from build123d import *

# Parameters (mm, degrees)
F0_R      = 1.5
F0_R_2    = 4.25
F1_DEPTH  = 3
F2_DEPTH  = 22
F3_W      = 9.5
F3_H      = 11
F2_FACE_W = 100
F2_FACE_H = 22
F4_DEPTH  = 50.001
F5_W      = 17
F5_H      = 3.3289747284
F6_DEPTH  = 76.9
F7_W      = 12.5
F7_H      = 8.2103219628
F7_H_2    = 8.3398447186
F7_H_3    = 8.5524427253
F8_DEPTH  = 63.2
F9_R      = 2
F10_DEPTH = 67.3


# Not quite as in the source:
# - a feature of the source that left no trace in its solid (it failed there, or was rolled back) is left out


with BuildPart() as f1:
    # F0 (on Top) → F1 (new body)
    with BuildSketch(Plane.XY):
        with BuildLine():
            Line((-48.5, -48.5), (0, -48.5))
            Line((0, -48.5), (0, -35.75))
            ThreePointArc((0, -35.75), (-4.25, -31.5), (0, -27.25))
            Line((0, -27.25), (0, -11.75))
            ThreePointArc((0, -11.75), (-4.25, -7.5), (0, -3.25))
            Line((0, -3.25), (0, 10.5))
            Line((0, 10.5), (-32, 10.5))
            Line((-32, 10.5), (-32, 26.5))
            Line((-32, 26.5), (0, 26.5))
            Line((0, 26.5), (0, 48.5))
            Line((0, 48.5), (-48.5, 48.5))
            Line((-48.5, 48.5), (-48.5, -48.5))
        make_face()
        with Locations((-32.5, -20.5)):
            Circle(F0_R, mode=Mode.SUBTRACT)
        with Locations((-32.5, -11.5)):
            Circle(F0_R, mode=Mode.SUBTRACT)
        with Locations((-32.5, -2.5)):
            Circle(F0_R, mode=Mode.SUBTRACT)
        with Locations((-14, -19.5)):
            Circle(F0_R_2, mode=Mode.SUBTRACT)
        with BuildLine():
            Line((0, -35.75), (0, -48.5))
            Line((0, -48.5), (48.5, -48.5))
            Line((48.5, -48.5), (48.5, 48.5))
            Line((48.5, 48.5), (0, 48.5))
            Line((0, 48.5), (0, 26.5))
            Line((0, 26.5), (32, 26.5))
            Line((32, 26.5), (32, 10.5))
            Line((32, 10.5), (0, 10.5))
            Line((0, 10.5), (0, -3.25))
            ThreePointArc((0, -3.25), (3.00520382, -4.49479618), (4.25, -7.5))
            ThreePointArc((4.25, -7.5), (3.00520382, -10.50520382), (0, -11.75))
            Line((0, -11.75), (0, -27.25))
            ThreePointArc((0, -27.25), (3.00520382, -28.49479618), (4.25, -31.5))
            ThreePointArc((4.25, -31.5), (3.00520382, -34.50520382), (0, -35.75))
        make_face()
        with Locations((14, -19.5)):
            Circle(F0_R_2, mode=Mode.SUBTRACT)
    extrude(amount=F1_DEPTH)

    # F0 (on Top) → F2 (join)
    with BuildSketch(Plane.XY):
        Polygon((50, 50), (-50, 50), (-50, -50), (0, -50), (50, -50), align=None)
        Polygon((48.5, -48.5), (0, -48.5), (-48.5, -48.5), (-48.5, 48.5), (0, 48.5), (48.5, 48.5), align=None, mode=Mode.SUBTRACT)
    extrude(amount=F2_DEPTH)

    # F3 (on Right) + F2_face (on face) → F4 (cut, through all)
    with BuildSketch(Plane.YZ):
        with Locations((-41.75, 25.5)):
            Rectangle(F3_W, F3_H)
    with BuildSketch(Plane(origin=(50, 0, 11), x_dir=(0, 1, 0), z_dir=(1, 0, 0))):
        Rectangle(F2_FACE_W, F2_FACE_H)
    extrude(amount=F4_DEPTH, mode=Mode.SUBTRACT)

    # F5 (on Right) → F6 (cut)
    with BuildSketch(Plane.YZ):
        with Locations((-22, 21.6644873642)):
            Rectangle(F5_W, F5_H)
    extrude(amount=F6_DEPTH, mode=Mode.SUBTRACT)

    # F7 (on Right) → F8 (cut)
    with BuildSketch(Plane.YZ):
        with Locations((32.75, 21.6051609814)):
            Rectangle(F7_W, F7_H)
        with Locations((15.25, 21.6699223593)):
            Rectangle(F7_W, F7_H_2)
        with Locations((-2.25, 21.7762213627)):
            Rectangle(F7_W, F7_H_3)
    extrude(amount=F8_DEPTH, mode=Mode.SUBTRACT)

    # F9 (on Right) → F10 (cut)
    with BuildSketch(Plane.YZ):
        with Locations((-12, 22)):
            Circle(F9_R)
        with Locations((-4, 22)):
            Circle(F9_R)
        with Locations((-20, 22)):
            Circle(F9_R)
        with Locations((-35.5, 22)):
            Circle(F9_R)
    extrude(amount=-F10_DEPTH, mode=Mode.SUBTRACT)


solid = f1.part
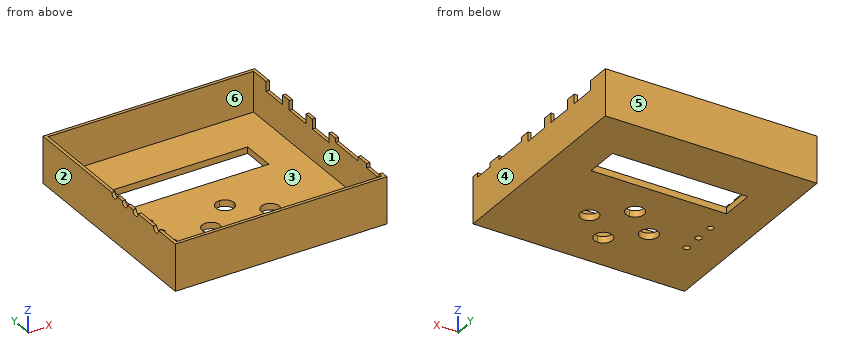
Model file for the job. Use its own axes, mm. Face numbers are marked on the shaded views. A direction names the side the tool comes from. Give positions to 0.01 mm unless a question says otherwise; leave off trailing zeros. Order: outer loops, then holes, each group sorted by start corner. A loop starts at its lowest first (then second) coordinate and runs counter-clockwise, first axis right, second up. Notation, with made-up numbers: (-10.5, 81) -> (27.5, 81) arc R20 cw to (27.5, 107) -> close; hole circle Ø8 at (0, 15.5). An arc over 180 degrees is marked (long way). Use CSV: the item, a comma, the result in double quotes.
1. Mould opens along X. For the marked faces 3, 4, 5 and 6 say: +X half, -X half, draft (parallel to the pull), parting line (faces both ways), or undercut.
Outcome:
face 3,"undercut"
face 4,"+X half"
face 5,"draft"
face 6,"undercut"
2. Band-saw the part on C-C, the plane y = 14. Give the cut face in (x, z).
Outcome:
outline,"(-50, 0) -> (-32, 0) -> (-32, 3) -> (-48.5, 3) -> (-48.5, 22) -> (-50, 22) -> close; (32, 0) -> (50, 0) -> (50, 17.5) -> (48.5, 17.5) -> (48.5, 3) -> (32, 3) -> close"
3. 3-axis set-ups, long thin cutter, end or side, ignore diameter. For the marked faces 1 and 2: which of +Z, -Z, +X, -X, +Y, -Y reach the whole face in a straight line?
Outcome:
face 1,"+Z"
face 2,"+Z, -Z, -X, +Y, -Y"
4. Band-saw the part on A-A, the plane x = -12. Give the cut face in (y, z).
Outcome:
outline,"(-50, 0) -> (-23.25, 0) -> (-23.25, 3) -> (-48.5, 3) -> (-48.5, 22) -> (-50, 22) -> close; (-15.75, 0) -> (10.5, 0) -> (10.5, 3) -> (-15.75, 3) -> close; (26.5, 0) -> (50, 0) -> (50, 22) -> (48.5, 22) -> (48.5, 3) -> (26.5, 3) -> close"
5. Drop flat-ended pins along their axis: pin 1 (0.8 mm diameter, centred on x = 49.5, y = -22, fed in from +Z); pin 2 (2.5 mm diameter, centred on x = -32.5, y = -11.5, fed in from -Z); pin 3 (1.2 mm diameter, centred on x = 49, y = -2.5, fed in from +Z); pin 4 (4 mm diameter, centred on x = -32.5, y = -20.5, fed in from +Z). Give the stop position or say it passes through.
Outcome:
pin 1,"z = 20"
pin 2,"through"
pin 3,"z = 17.5"
pin 4,"z = 3"
6. Band-saw the part on B-B, the plane z = 6.5. Give the cut face in (x, y).
Outcome:
outline,"(-50, -50) -> (50, -50) -> (50, 50) -> (-50, 50) -> close; hole (-48.5, -48.5) -> (48.5, -48.5) -> (48.5, 48.5) -> (-48.5, 48.5) -> close"
7. Band-saw the part on D-D, the plane x = 26. Give the cut face in (y, z).
Outcome:
outline,"(-50, 0) -> (10.5, 0) -> (10.5, 3) -> (-48.5, 3) -> (-48.5, 22) -> (-50, 22) -> close; (26.5, 0) -> (50, 0) -> (50, 22) -> (48.5, 22) -> (48.5, 3) -> (26.5, 3) -> close"
8. Drill centre lines: line 1 along Y through (x, z) = (14, 0.8); line 2 along X through (y, z) = (-32.5, 10.75). Where is each one in solid material? Low to high. Write a range as from..to.
Outcome:
line 1,"-50..-23.75, -15.25..10.5, 26.5..50"
line 2,"-50..-48.5, 48.5..50"
